Input: part model. Units: mm. Frame: model coordinates. A direction names the side the tool comes from. Coordinates: 2 decimals unless noted, no trailing zeros. Loops run counter-clockwise (first coordinate to the right, second up) from the corner with the lowest first, then second, coordinate; pieces in that order, holes last.
(1) Section C-C, the plane y = 2.75. Return loops of the section in (x, z), then the cut area to 3 significant figures.
(2) Line query: L1, parallel to X at y = 13.25, z = 2.5; L2, parallel to X at y = 3, z = 28; L3, parallel to Z at x = 28, y = 7.5. Output: solid intervals per line, ascending.
(3) Contact query for flat-ended pins moving along their axis: P1, Ø5.5, axis at x = -34, y = 12.5, coming from the -Z side; P2, Ø5.5, axis at y = 13, z = -35, coming from the -X side; P3, Ø6, axis at y = 15, z = 9, coming from the -X side. Output: stop coordinate, or through.
(4) Set-up query: faces 4 (the face through (-34, 16, -1.65)), 5 (the face through (-25, 17.5, 25)), 6 (the face through (-25, 17.5, -25)). Return all of +Z, -Z, +X, -X, +Y, -Y with unobstructed straight access to the full face (end or side cutting, diameter ignored); none if empty.
(5) Section D-D, the plane y = 12. Return loops of the section in (x, z).
(6) Section B-B, the plane x = 16. Return loops of the section in (y, z), then the cut area to 3 significant figures.
(7) Mould query, pull axis Z, two halves, no side actions, for faces 1 (the face through (22, 20, 25)), 2 (the face through (40.21, 2.54, 0.38)), 3 (the face through (26.065, 18.768, 26.612)). Classes: released by +Z, released by -Z, zero draft, split by the parting line, or undercut.
(8) Section A-A, the plane z = 0. Return loops of the section in (x, y).
```python
from build123d import *

# Parameters (mm, degrees)
CUT_EXTRUDE1_DEPTH = 64.679863379
CIRPATTERN1_COUNT  = 4
SKETCH4_R          = 1.75
CUT_EXTRUDE2_DEPTH = 10
CIRPATTERN2_COUNT  = 6


with BuildPart() as part:
    # Sketch2 → Revolve1 (revolve)
    with BuildSketch(Plane.XY, mode=Mode.PRIVATE) as revolve1_sk:
        Polygon((-32.25, 20), (-32.25, 0), (-42.75, 0), (-42.75, 5), (-34.75, 5), (-34.75, 17.5), (-37.25, 17.5), (-37.25, 20), align=None)
    revolve(revolve1_sk.sketch.rotate(Axis((0, 0, 0), (0, 1, 0)), 270), axis=Axis((0, 0, 0), (0, 1, 0)))

    # Sketch3 → Cut-Extrude1 (cut, symmetric)
    with BuildSketch(Plane(origin=(0, 0, 0), x_dir=(0, 0, -1), z_dir=(1, 0, 0))):
        with BuildLine():
            Line((-1.65, 29.999999659), (1.65, 29.999999659))
            Line((1.65, 29.999999659), (1.65, 10.000000341))
            ThreePointArc((1.65, 10.000000341), (0, 8.35), (-1.65, 10.000000341))
            Line((-1.65, 10.000000341), (-1.65, 29.999999659))
        make_face()
    cut_extrude1 = extrude(amount=CUT_EXTRUDE1_DEPTH, both=True, mode=Mode.SUBTRACT)

    # CirPattern1: Cut-Extrude1 ×4 about axis
    cirpattern1_axis = Axis((0, 0, 0), (0, -1, 0))
    for i in range(1, CIRPATTERN1_COUNT):
        add(cut_extrude1.rotate(cirpattern1_axis, i * 360 / CIRPATTERN1_COUNT), mode=Mode.SUBTRACT)

    # Sketch4 → Cut-Extrude2 (cut)
    with BuildSketch(Plane(origin=(0, 5, 0), x_dir=(1, 0, 0), z_dir=(0, 1, 0))):
        with Locations(Location((-38.5, 0, 0), (0, 0, 270))):
            Circle(SKETCH4_R)
    cut_extrude2 = extrude(amount=-CUT_EXTRUDE2_DEPTH, mode=Mode.SUBTRACT)

    # CirPattern2: Cut-Extrude2 ×6 about axis
    cirpattern2_axis = Axis((0, 0, 0), (0, 1, 0))
    for i in range(1, CIRPATTERN2_COUNT):
        add(cut_extrude2.rotate(cirpattern2_axis, i * 360 / CIRPATTERN2_COUNT), mode=Mode.SUBTRACT)


solid = part.part
```
Report:
1. outline: circle Ø85.5 at (0, 0); hole circle Ø3.5 at (-38.5, 0); hole circle Ø64.5 at (0, 0); hole circle Ø3.5 at (-19.25, -33.34); hole circle Ø3.5 at (-19.25, 33.34); hole circle Ø3.5 at (19.25, -33.34); hole circle Ø3.5 at (19.25, 33.34); hole circle Ø3.5 at (38.5, 0)
1. area: 2,420 mm2
2. L1: x = -34.66 to -32.15, 32.15 to 34.66
2. L2: x = -32.3 to -16, 16 to 32.3
2. L3: z = -20.58 to -16, 16 to 20.58
3. P1: stops at z = -15.2
3. P2: stops at x = -12.94
3. P3: stops at x = -36.52
4. face 4: +X, -X, +Y
4. face 5: +Z, -X
4. face 6: -Z, -X
5. outline: (-34.71, -1.65) arc R34.75 ccw to (-1.65, -34.71) - (-1.65, -32.21) arc R32.25 cw to (-32.21, -1.65) - close; (-34.71, 1.65) - (-32.21, 1.65) arc R32.25 cw to (-1.65, 32.21) - (-1.65, 34.71) arc R34.75 ccw to start; (1.65, -34.71) arc R34.75 ccw to (34.71, -1.65) - (32.21, -1.65) arc R32.25 cw to (1.65, -32.21) - close; (1.65, 32.21) arc R32.25 cw to (32.21, 1.65) - (34.71, 1.65) arc R34.75 ccw to (1.65, 34.71) - close
6. outline: (0, -39.64) - (5, -39.64) - (5, -30.85) - (17.5, -30.85) - (17.5, -33.64) - (20, -33.64) - (20, -28) - (0, -28) - close; (0, 28) - (20, 28) - (20, 33.64) - (17.5, 33.64) - (17.5, 30.85) - (5, 30.85) - (5, 39.64) - (0, 39.64) - close
6. area: 216 mm2
7. face 1: zero draft
7. face 2: undercut
7. face 3: released by +Z
8. outline: (-42.75, 0) - (-40.25, 0) - (-40.25, 5) - (-42.75, 5) - close; (-36.75, 0) - (-32.25, 0) - (-32.25, 8.35) - (-34.75, 8.35) - (-34.75, 5) - (-36.75, 5) - close; (32.25, 0) - (36.75, 0) - (36.75, 5) - (34.75, 5) - (34.75, 8.35) - (32.25, 8.35) - close; (40.25, 0) - (42.75, 0) - (42.75, 5) - (40.25, 5) - close
